Check sheet for the drawn part. Datum: minimum x, y, z corner. Units: mm. A direction names the side the tool comes from. Round coordinates to 2 decimals unless told otherwise and drop trailing zeros. Loops run counter-clockwise (first coordinate to the right, second up) from the corner with the lowest first, then second, coordinate; pieces in that order, holes last. Notation, with made-up numbers: (57, -33.75) -> (106, -33.75) arc R15 ccw to (106, -14.75) -> close; hole circle Ø7 at (89, 61). An arc over 180 degrees is marked (long way). Return JSON: item names as keys, results as strings.
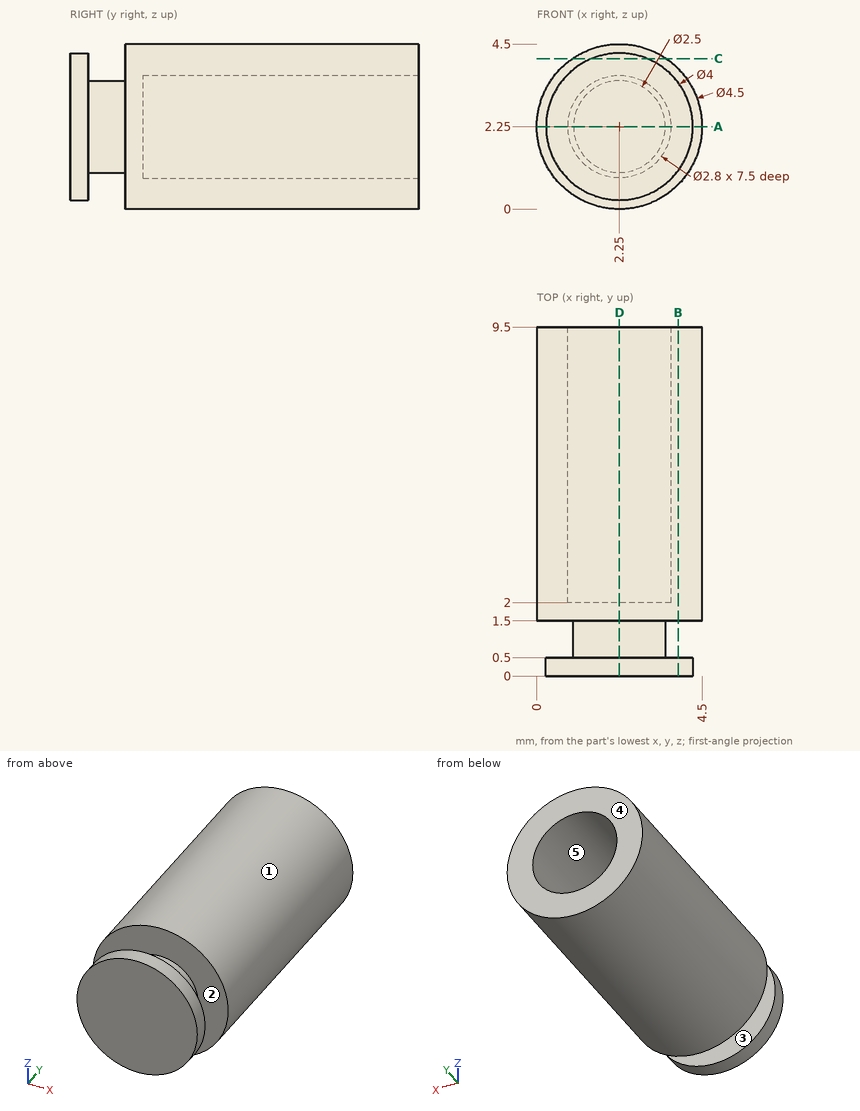
Q1. Section check A-A (z = 2.25). Record the boundary of the cut face in (x, y), then the cut area to 3 significant figures.
Results list:
{"outline": "(0, 1.5) -> (1, 1.5) -> (1, 0.5) -> (0.25, 0.5) -> (0.25, 0) -> (4.25, 0) -> (4.25, 0.5) -> (3.5, 0.5) -> (3.5, 1.5) -> (4.5, 1.5) -> (4.5, 9.5) -> (3.65, 9.5) -> (3.65, 2) -> (0.85, 2) -> (0.85, 9.5) -> (0, 9.5) -> close", "area": "19.5 mm^2"}
Q2. Go/stop test with flat-tipped pins: pin 1 (1 mm diameter, centred on x = 1, z = 2, fed in from +Y); pin 2 (1 mm diameter, centred on x = 3, z = 2, fed in from +Y). Record where each tip stops, or that it passes through.
Results list:
{"pin 1": "y = 9.5", "pin 2": "y = 2"}
Q3. Tool access check on the marked faces 1 and 2. Record the directions out of +Z, -Z, +X, -X, +Y, -Y that give a thin tool (end or side, any length) a straight path to the whole face; none if there is none.
Results list:
{"face 1": "+Y, -Y", "face 2": "none"}
Q4. Material ranges on line 1 (X direction, y = 5.75, z = 2.25); line 2 (Y direction, x = 3.95, z = 1.45), recorded low to high.
Results list:
{"line 1": "0 to 0.85, 3.65 to 4.5", "line 2": "0 to 0.5, 1.5 to 9.5"}
Q5. Section check C-C (z = 4.1). Record the boundary of the cut face in (x, y).
Results list:
{"outline": "(0.97, 1.5) -> (3.53, 1.5) -> (3.53, 9.5) -> (0.97, 9.5) -> close; (1.49, 0) -> (3.01, 0) -> (3.01, 0.5) -> (1.49, 0.5) -> close"}
Q6. Section check D-D (x = 2.25). Record the boundary of the cut face in (y, z), then the cut area to 3 significant figures.
Results list:
{"outline": "(0, 0.25) -> (0.5, 0.25) -> (0.5, 1) -> (1.5, 1) -> (1.5, 0) -> (9.5, 0) -> (9.5, 0.85) -> (2, 0.85) -> (2, 3.65) -> (9.5, 3.65) -> (9.5, 4.5) -> (1.5, 4.5) -> (1.5, 3.5) -> (0.5, 3.5) -> (0.5, 4.25) -> (0, 4.25) -> close", "area": "19.5 mm^2"}
Q7. Draft check along Y on the marked faces 3, 4 and 5. Enter one of: released by +Y, released by -Y, zero draft, split by the parting line, or undercut.
Results list:
{"face 3": "undercut", "face 4": "released by +Y", "face 5": "zero draft"}
Q8. Section check B-B (x = 3.85). Record the boundary of the cut face in (y, z), then the cut area to 3 significant figures.
Results list:
{"outline": "(0, 1.05) -> (0.5, 1.05) -> (0.5, 3.45) -> (0, 3.45) -> close; (1.5, 0.67) -> (9.5, 0.67) -> (9.5, 3.83) -> (1.5, 3.83) -> close", "area": "26.5 mm^2"}
